Here's how the part is built. I have some questions about the finished solid (model axes, mm). Face numbers are marked on the shaded views. A direction names the side the tool comes from. Round coordinates to 2 decimals unless told otherwise and drop trailing zeros. Write each loop counter-clockwise with the first axis right and the second up, starting at its lowest first coordinate (ties: lowest second). Pieces come first, ordered by that corner, then holes. Notation, with made-up numbers: (-13, 72) -> (46, 72) arc R17 ccw to (46, 99) -> close; hole circle Ø4 at (67, -37.5). An arc over 180 degrees is marked (long way). Answer as CSV lines item,"result".
```python
from build123d import *

# Parameters (mm, degrees)
IZIM1_W                     = 64
IZIM1_H                     = 64
Y_KSEKLIK_EKSTR_ZYON1_DEPTH = 10
IZIM2_W                     = 36
IZIM2_H                     = 36
Y_KSEKLIK_EKSTR_ZYON2_DEPTH = 28
IZIM3_R                     = 3
KES_EKSTR_ZYON1_DEPTH       = 20
IZIM4_R                     = 3
KES_EKSTR_ZYON2_DEPTH       = 20
IZIM5_R                     = 3
KES_EKSTR_ZYON3_DEPTH       = 11


with BuildPart() as part:
    # Çizim1 → Yükseklik-Ekstrüzyon1 (new body)
    with BuildSketch(Plane.XY):
        with Locations((-32, -32)):
            Rectangle(IZIM1_W, IZIM1_H)
    extrude(amount=Y_KSEKLIK_EKSTR_ZYON1_DEPTH)

    # Çizim2 → Yükseklik-Ekstrüzyon2 (add)
    with BuildSketch(Plane.XY.offset(10)):
        with Locations((-46, -18)):
            Rectangle(IZIM2_W, IZIM2_H)
    extrude(amount=Y_KSEKLIK_EKSTR_ZYON2_DEPTH)

    # Çizim3 → Kes-Ekstrüzyon1 (cut)
    with BuildSketch(Plane.XZ.offset(36)):
        with Locations((-42, 24)):
            Circle(IZIM3_R)
    extrude(amount=-KES_EKSTR_ZYON1_DEPTH, mode=Mode.SUBTRACT)

    # Çizim4 → Kes-Ekstrüzyon2 (cut)
    with BuildSketch(Plane(origin=(-28, 0, 0), x_dir=(0, 0, -1), z_dir=(1, 0, 0))):
        with Locations((-24, -22)):
            Circle(IZIM4_R)
    extrude(amount=-KES_EKSTR_ZYON2_DEPTH, mode=Mode.SUBTRACT)

    # Çizim5 → Kes-Ekstrüzyon3 (cut, through all)
    with BuildSketch(Plane.XY.offset(10)):
        with Locations((-14, -50)):
            Circle(IZIM5_R)
        with Locations((-14, -12)):
            Circle(IZIM5_R)
        with Locations((-52, -50)):
            Circle(IZIM5_R)
    extrude(amount=-KES_EKSTR_ZYON3_DEPTH, mode=Mode.SUBTRACT)


solid = part.part
```
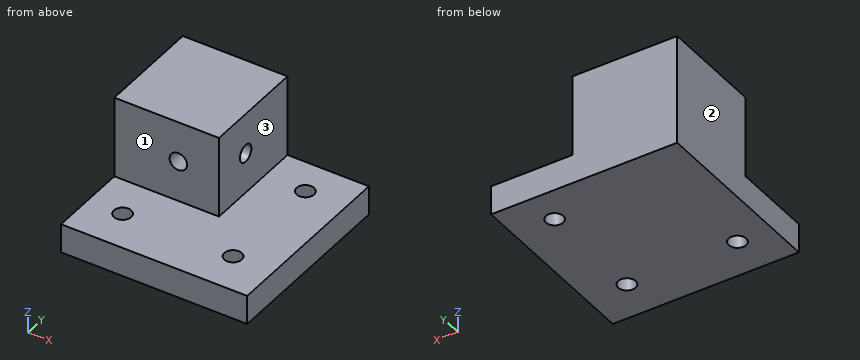
1. For pin 1 Ø2 at (x, y) = (-6.5, -10) entering from -Z; pin 2 Ø3.5 at (x, y) = (-14, -50) entering from +Z; pin 3 Ø7 at (x, y) = (-52, -50) entering from +Z; pin 4 Ø8.5 at (y, z) = (-11.5, 29.5) entering from +X, each with a flat end and sliding along its axis, tell me the tip position at first contact or that it passes through.
Numbers:
pin 1,"stops at z = 0"
pin 2,"passes through"
pin 3,"stops at z = 10"
pin 4,"stops at x = -28"
2. Suppose I cut it at B-B on x = -31.5. Please give me the cut outline in (y, z).
Numbers:
outline,"(-64, 0) -> (0, 0) -> (0, 38) -> (-36, 38) -> (-36, 10) -> (-64, 10) -> close; hole circle Ø6 at (-22, 24)"
3. If I drill on line 1 (Z direction, x = -34.25, y = -22); line 2 (Z direction, x = -6.5, y = -11.5); line 3 (X direction, y = -24, z = 16), over which ranges is the centre line in solid material (lowest first)?
Numbers:
line 1,"z = 0 to 21, 27 to 38"
line 2,"z = 0 to 10"
line 3,"x = -64 to -28"
4. Suppose I cut it at D-D on z = 9. Please give me the cut outline in (x, y), and give its area (3 significant figures).
Numbers:
outline,"(-64, -64) -> (0, -64) -> (0, 0) -> (-64, 0) -> close; hole circle Ø6 at (-52, -50); hole circle Ø6 at (-14, -50); hole circle Ø6 at (-14, -12)"
area,"4,010 mm^2"
5. On a 3-axis mill with a long thin cutter (end or side, diameter ignored), from which of +Z, -Z, +X, -X, +Y, -Y can I reach the whole of each face in a straight line? I mean the marked faces 1, 2 and 3. Say none if no direction works.
Numbers:
face 1,"+Z, +X, -X, -Y"
face 2,"+Z, -Z, -X, +Y, -Y"
face 3,"+Z, +X, +Y, -Y"
6. Suppose I cut it at C-C on y = -29. Please give me the cut outline in (x, z), and give its area (3 significant figures).
Numbers:
outline,"(-64, 0) -> (0, 0) -> (0, 10) -> (-28, 10) -> (-28, 38) -> (-64, 38) -> close; hole circle Ø6 at (-42, 24)"
area,"1,620 mm^2"
7. Suppose I cut it at A-A on x = -14. Please give me the cut outline in (y, z), and give its area (3 significant figures).
Numbers:
outline,"(-64, 0) -> (-53, 0) -> (-53, 10) -> (-64, 10) -> close; (-47, 0) -> (-15, 0) -> (-15, 10) -> (-47, 10) -> close; (-9, 0) -> (0, 0) -> (0, 10) -> (-9, 10) -> close"
area,"520 mm^2"
